Geometry check sheet. Reference: drawing and pictorial views, mm from the part's lowest x, y, z. A direction names the side the tool comes from. Coordinates: 2 decimals unless noted, no trailing zeros. Loops run counter-clockwise (first coordinate to the right, second up) from the corner with the lowest first, then second, coordinate; pieces in that order, holes last. Notation, with made-up numbers: (80, 19.5) - (112, 19.5) arc R18 cw to (112, 53.5) - close; hole circle Ø9 at (22, 70.5). An arc over 180 degrees is marked (long way). Write each question's results on one line, items separated by ' | '. Start each with the question number.
1. Thickness scan on line 1 (Z direction, x = 16, y = 8); line 2 (X direction, y = 3.75, z = 6); line 3 (X direction, y = 7.75, z = 4.75). Record the ranges inside material, lowest first. Write a range as [from, to].
2. Cross-section at D-D (y = 9.5). Record the cut outline in (x, z).
3. Tool access check on the marked faces 1 and 2. Record the directions out of +Z, -Z, +X, -X, +Y, -Y that give a thin tool (end or side, any length) a straight path to the whole face; none if there is none.
4. Cross-section at A-A (z = 3.75). Record the cut outline in (x, y).
5. Cross-section at C-C (y = 5). Record the cut outline in (x, z).
6. Cross-section at B-B (x = 11). Record the cut outline in (y, z).
7. Draft check along X on the marked faces 3 and 4. Enter one of: released by +X, released by -X, zero draft, split by the parting line, or undercut.
8. Gauge pin test, flat ends, axial feed: P1, Ø4, axis at y = 5, z = 4.5, coming from the -X side; P2, Ø6, axis at x = 17, y = 1.5, coming from the +Z side; P3, Ø1.5, axis at x = 33.5, y = 6, coming from the -Z side; P4, Ø1.5, axis at y = 9, z = 3, coming from the +X side. Record the tip position at first contact, or that the pin passes through.
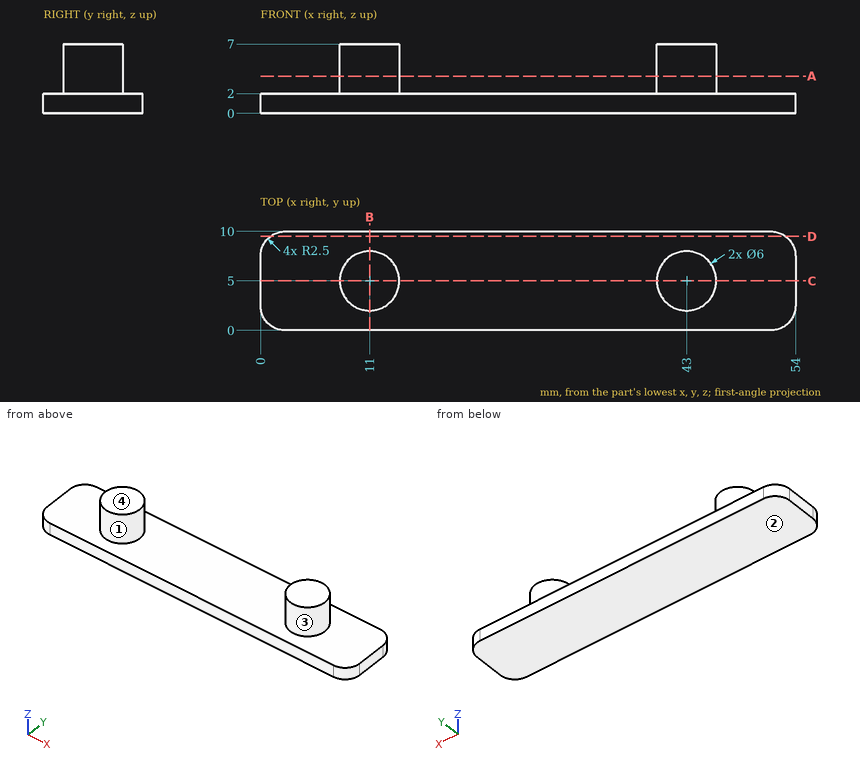
Established:
1) line 1: [0, 2] | line 2: [8.27, 13.73], [40.27, 45.73] | line 3: [9.8, 12.2], [41.8, 44.2]
2) outline: (1, 0) - (53, 0) - (53, 2) - (1, 2) - close
3) face 1: +Z | face 2: -Z, +X, -X, +Y, -Y
4) outline: circle Ø6 at (11, 5); circle Ø6 at (43, 5)
5) outline: (0, 0) - (54, 0) - (54, 2) - (46, 2) - (46, 7) - (40, 7) - (40, 2) - (14, 2) - (14, 7) - (8, 7) - (8, 2) - (0, 2) - close
6) outline: (0, 0) - (10, 0) - (10, 2) - (8, 2) - (8, 7) - (2, 7) - (2, 2) - (0, 2) - close
7) face 3: undercut | face 4: zero draft
8) P1: x = 8 | P2: z = 2 | P3: z = 0 | P4: through
